Part model, mm, in its own coordinate system. Face numbers are marked on the shaded views. A direction names the side the tool comes from. Round coordinates to 2 decimals unless told otherwise and drop trailing zeros. Write each loop counter-clockwise with the first axis right and the second up, starting at its lowest first coordinate (ties: lowest second). Pieces come first, ordered by that corner, then holes.
1) Saw through at B-B on y = -14.5. Write the cut outline in (x, z).
2) Saw through at D-D on z = 29.4. Write the cut outline in (x, y), and give its area (3 significant figures).
3) Flat gauge pins, fed straight in: pin 1 (10 mm diameter, centred on y = -9.5, z = 9.5, fed in from +X); pin 2 (5.5 mm diameter, centred on y = -14.5, z = 29.4, fed in from -X); pin 3 (8 mm diameter, centred on x = 3, z = -8.5, fed in from +Y); pin 4 (12 mm diameter, centred on x = 18, y = -16, fed in from +Z). Where does each tip first touch, or does it go through?
4) Pull direction X, two halves, no side cores. Call the marked faces 3, 4 and 5: +X half, -X half, draft (parallel to the pull), parting line (faces both ways), or undercut.
5) Saw through at A-A on z = 51.7. Write the cut outline in (x, y), and give its area (3 significant figures).
6) Drill centre lines: L1, parallel to Y at x = 1.3, z = 51.7; L2, parallel to Y at x = 19.5, z = 32.5; L3, parallel to X at y = -9.25, z = 48.5. Where is each one in solid material? Low to high.
7) Which spindle directions (+Z, -Z, +X, -X, +Y, -Y) get a long thin tool onto all of the face, cutting with end or side? Do the marked faces 1 and 2. Say none if no direction does.
8) Saw through at C-C on x = 22. Write the cut outline in (y, z), and give its area (3 significant figures).
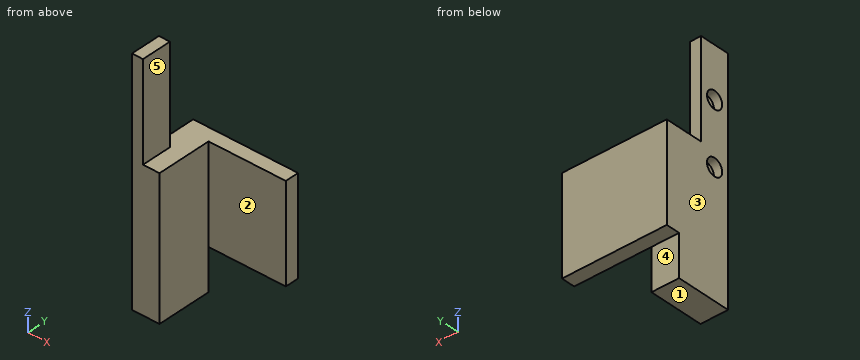
```python
from build123d import *

# Parameters (mm, degrees)
SKETCH_1_W          = 38
SKETCH_1_H          = 35
EXTRUDE_1_DEPTH     = 5
SKETCH_1_14_W       = 10
SKETCH_1_14_H       = 50
EXTRUDE_2_DEPTH     = 20
EXTRUDE_START       = -10
SKETCH_2_W          = 35
SKETCH_2_H          = 11
EXTRUDE_3_DEPTH     = 4
CUT_EXTRUDE_START   = -10
SKETCH_2_3_R        = 3.1
CUT_EXTRUDE_1_DEPTH = 3


with BuildPart() as part:
    # 草图1 → 凸台-拉伸1 (new body)
    with BuildSketch(Plane(origin=(0, 0, 0), x_dir=(1, 0, 0), z_dir=(0, 1, 0))):
        with Locations((19, -17.5)):
            Rectangle(SKETCH_1_W, SKETCH_1_H)
    extrude(amount=EXTRUDE_1_DEPTH)

    # 草图1<14> → 凸台-拉伸2 (add)
    with BuildSketch(Plane(origin=(0, 0, 0), x_dir=(1, 0, 0), z_dir=(0, 1, 0))):
        with Locations((5, -10)):
            Rectangle(SKETCH_1_14_W, SKETCH_1_14_H)
    extrude(amount=-EXTRUDE_2_DEPTH)

    # 草图2 → 凸台-拉伸3 (add)
    with BuildSketch(Plane(origin=(10, 0, 0), x_dir=(0, 0, -1), z_dir=(1, 0, 0)).offset(EXTRUDE_START)):
        with Locations((-52.5, -14.5)):
            Rectangle(SKETCH_2_W, SKETCH_2_H)
    extrude(amount=EXTRUDE_3_DEPTH)

    # 草图2<3> → 切除-拉伸1 (cut)
    with BuildSketch(Plane(origin=(10, 0, 0), x_dir=(0, 0, -1), z_dir=(1, 0, 0)).offset(CUT_EXTRUDE_START)):
        with Locations((-29.4, -14.5)):
            Circle(SKETCH_2_3_R)
        with Locations((-51.7, -14.5)):
            Circle(SKETCH_2_3_R)
    extrude(amount=CUT_EXTRUDE_1_DEPTH, mode=Mode.SUBTRACT)


solid = part.part
```
Completed:
1. outline: (0, -15) - (10, -15) - (10, 35) - (4, 35) - (4, 70) - (0, 70) - (0, 54.8) - (3, 54.8) - (3, 48.6) - (0, 48.6) - (0, 32.5) - (3, 32.5) - (3, 26.3) - (0, 26.3) - close
2. outline: (0, -20) - (10, -20) - (10, 0) - (38, 0) - (38, 5) - (0, 5) - (0, -11.4) - (3, -11.4) - (3, -17.6) - (0, -17.6) - close
2. area: 371 mm2
3. pin 1: stops at x = 10
3. pin 2: stops at x = 3
3. pin 3: stops at y = 0
3. pin 4: passes through
4. face 3: -X half
4. face 4: draft
4. face 5: +X half
5. outline: (0, -20) - (4, -20) - (4, -9) - (0, -9) - (0, -11.4) - (3, -11.4) - (3, -17.6) - (0, -17.6) - close
5. area: 25.4 mm2
6. L1: y = -20 to -17.6, -11.4 to -9
6. L2: y = 0 to 5
6. L3: x = 0 to 4
7. face 1: -Z, +X, -X, +Y, -Y
7. face 2: +Z, -Z, +X, -Y
8. outline: (0, 0) - (5, 0) - (5, 35) - (0, 35) - close
8. area: 175 mm2
